from build123d import *

# Parameters (mm, degrees)
F1_DEPTH = 40
F2_DEPTH = 46
F4_DEPTH = 27
F5_DEPTH = 60.6


with BuildPart() as f1:
    # F0 (on Top) → F1 (new body, symmetric)
    with BuildSketch(Plane.XY):
        with BuildLine():
            Line((-49, 0), (0, 0))
            Line((0, 0), (41, 0))
            Line((41, 0), (41, 10))
            Line((41, 10), (42.9, 10))
            Line((42.9, 10), (49, 10))
            ThreePointArc((49, 10), (43.3431457505, 12.3431457505), (41, 18))
            Line((41, 18), (41, 19.9))
            Line((41, 19.9), (0, 19.9))
            Line((0, 19.9), (-41, 19.9))
            Line((-41, 19.9), (-41, 18))
            ThreePointArc((-41, 18), (-43.3431457505, 12.3431457505), (-49, 10))
            Line((-49, 10), (-49, 9.95))
            Line((-49, 9.95), (-49, 0))
        make_face()
        Polygon((41, 0), (0, 0), (-49, 0), (-49, -15), (0, -15), (41, -15), align=None)
        with BuildLine():
            Line((41, 10), (41, 0))
            Line((41, 0), (41, -15))
            Line((41, -15), (63.5, -15))
            ThreePointArc((63.5, -15), (51, -2.5), (63.5, 10))
            Line((63.5, 10), (49, 10))
            Line((49, 10), (42.9, 10))
            Line((42.9, 10), (41, 10))
        make_face()
        with BuildLine():
            ThreePointArc((76, -2.5), (72.3388347648, -11.3388347648), (63.5, -15))
            Line((63.5, -15), (86, -15))
            Line((86, -15), (86, -2.5))
            Line((86, -2.5), (86, 10))
            Line((86, 10), (63.5, 10))
            ThreePointArc((63.5, 10), (72.3388347648, 6.3388347648), (76, -2.5))
        make_face()
        Polygon((86, -2.5), (86, -15), (131, -15), (131, 10), (86, 10), align=None)
        with BuildLine():
            Line((63.5, -2.5), (63.5, -13.5))
            ThreePointArc((63.5, -13.5), (71.2781745931, -10.2781745931), (74.5, -2.5))
            ThreePointArc((74.5, -2.5), (71.2781745931, 5.2781745931), (63.5, 8.5))
            Line((63.5, 8.5), (63.5, -2.5))
        make_face()
        with BuildLine():
            ThreePointArc((63.5, 8.5), (52.5, -2.5), (63.5, -13.5))
            Line((63.5, -13.5), (63.5, -2.5))
            Line((63.5, -2.5), (63.5, 8.5))
        make_face()
        with BuildLine():
            ThreePointArc((63.5, 10), (51, -2.5), (63.5, -15))
            Line((63.5, -15), (63.5, -13.5))
            ThreePointArc((63.5, -13.5), (52.5, -2.5), (63.5, 8.5))
            Line((63.5, 8.5), (63.5, 10))
        make_face()
        with BuildLine():
            Line((63.5, -13.5), (63.5, -15))
            ThreePointArc((63.5, -15), (72.3388347648, -11.3388347648), (76, -2.5))
            ThreePointArc((76, -2.5), (72.3388347648, 6.3388347648), (63.5, 10))
            Line((63.5, 10), (63.5, 8.5))
            ThreePointArc((63.5, 8.5), (71.2781745931, 5.2781745931), (74.5, -2.5))
            ThreePointArc((74.5, -2.5), (71.2781745931, -10.2781745931), (63.5, -13.5))
        make_face()
    extrude(amount=F1_DEPTH, both=True)

    # F0 (on Top) → F2 (join)
    with BuildSketch(Plane.XY):
        with BuildLine():
            ThreePointArc((63.5, 10), (51, -2.5), (63.5, -15))
            Line((63.5, -15), (63.5, -13.5))
            ThreePointArc((63.5, -13.5), (52.5, -2.5), (63.5, 8.5))
            Line((63.5, 8.5), (63.5, 10))
        make_face()
        with BuildLine():
            Line((63.5, -13.5), (63.5, -15))
            ThreePointArc((63.5, -15), (72.3388347648, -11.3388347648), (76, -2.5))
            ThreePointArc((76, -2.5), (72.3388347648, 6.3388347648), (63.5, 10))
            Line((63.5, 10), (63.5, 8.5))
            ThreePointArc((63.5, 8.5), (71.2781745931, 5.2781745931), (74.5, -2.5))
            ThreePointArc((74.5, -2.5), (71.2781745931, -10.2781745931), (63.5, -13.5))
        make_face()
    extrude(amount=F2_DEPTH)

    # F3 (on face) → F4 (cut)
    with BuildSketch(Plane(origin=(0, 19.9, 0), x_dir=(-1, 0, 0), z_dir=(0, 1, 0))):
        Polygon((-33, 0), (-28, 0), (-28, 28), (0, 28), (0, 33), (-33, 33), align=None)
        Polygon((28, 28), (28, 0), (28, -28), (0, -28), (-28, -28), (-28, 0), (-33, 0), (-33, -33), (0, -33), (33, -33), (33, 0), (33, 33), (0, 33), (0, 28), align=None)
    extrude(amount=-F4_DEPTH, mode=Mode.SUBTRACT)

    # F5 (cut): a face of the model
    f5_faces = [f1.faces().sort_by_distance(p)[0] for p in [
        (0, 19.9, 0),
    ]]
    extrude(f5_faces, amount=-F5_DEPTH, mode=Mode.SUBTRACT)


solid = f1.part
Part model, mm, in its own coordinate system. A direction names the side the tool comes from. Round coordinates to 2 decimals unless told otherwise and drop trailing zeros. Write each loop counter-clockwise with the first axis right and the second up, starting at its lowest first coordinate (ties: lowest second). Pieces come first, ordered by that corner, then holes. Notation, with made-up numbers: (21.5, 61.5) - (38.5, 61.5) arc R21 ccw to (38.5, 83.5) - close; hole circle Ø2 at (32.5, 0). An arc over 180 degrees is marked (long way). Use CSV: the item, a comma, the result in double quotes.
Item 1: Flat gauge pins, fed straight in: P1, Ø2, axis at x = 93.5, z = -31, coming from the +Y side; P2, Ø8, axis at y = 13, z = -9.5, coming from the -X side; P3, Ø7.5, axis at x = 100.5, y = -8.5, coming from the +Z side; P4, Ø0.6, axis at y = 19, z = 9.5, coming from the +X side. Where does each tip first touch, or does it go through?
Results list:
P1,"stops at y = 10"
P2,"stops at x = -49"
P3,"stops at z = 40"
P4,"stops at x = 41"
Item 2: Slice it at B-B, the plane y = -10.5. Write the cut outline in (x, z), then the cut area to 3 significant figures.
Results list:
outline,"(-49, -40) - (131, -40) - (131, 40) - (73.1, 40) - (73.1, 46) - (71.05, 46) - (71.05, 40) - (55.95, 40) - (55.95, 46) - (53.9, 46) - (53.9, 40) - (-49, 40) - close; hole (-28, -28) - (28, -28) - (28, 28) - (-28, 28) - close"
area,"11,300 mm²"
Item 3: Wall check: L1, parallel to X at y = -12.5, z = 10.5; L2, parallel to Z at x = 8, y = 7; L3, parallel to X at y = 1, z = -5. Give the ranges that are in metal, low to high.
Results list:
L1,"x = -49 to -28, 28 to 131"
L2,"z = -40 to -33, 33 to 40"
L3,"x = -49 to -33, 33 to 131"
Item 4: Slice it at A-A, the plane z = -12. Write the cut outline in (x, y).
Results list:
outline,"(-49, -15) - (-28, -15) - (-28, -7.1) - (-33, -7.1) - (-33, 19.9) - (-41, 19.9) - (-41, 18) arc R8 cw to (-49, 10) - close; (28, -15) - (131, -15) - (131, 10) - (49, 10) arc R8 cw to (41, 18) - (41, 19.9) - (33, 19.9) - (33, -7.1) - (28, -7.1) - close"
Item 5: Slice it at C-C, the plane x = 103.5. Write the cut outline in (y, z), then the cut area to 3 significant figures.
Results list:
outline,"(-15, -40) - (10, -40) - (10, 40) - (-15, 40) - close"
area,"2,000 mm²"
Item 6: Slice it at D-D, the plane y = 4.5. Write the cut outline in (x, z), then the cut area to 3 significant figures.
Results list:
outline,"(-49, -40) - (131, -40) - (131, 40) - (73.86, 40) - (73.86, 46) - (71.99, 46) - (71.99, 40) - (55.01, 40) - (55.01, 46) - (53.14, 46) - (53.14, 40) - (-49, 40) - close; hole (-33, -33) - (33, -33) - (33, 33) - (-33, 33) - close"
area,"10,100 mm²"
Item 7: Pull direction Z, two halves, no side cores. Call faces 1 (the flat face through (1, 19.9, -35)), 2 (the flat face through (104, -2, 40)), 3 (the flat face through (0, -11, 28)): pulls with the +Z half, pulls with the -Z half, needs draft (parallel to the pull), parting line crosses it, or undercut.
Results list:
face 1,"needs draft"
face 2,"pulls with the +Z half"
face 3,"undercut"
Item 8: Tool access for faces 4 (the flat face through (0, -11, -28)), 5 (the flat face through (-49, -2, 1)), 6 (the flat face through (91, 10, 1)), 7 (the flat face through (63, -2, 40)), 8 (the flat face through (0, 7, -33)): list every direction of +Z, -Z, +X, -X, +Y, -Y with a clear straight run to the whole face (end or side of a thin tool).
Results list:
face 4,"+Y, -Y"
face 5,"+Z, -Z, -X, +Y, -Y"
face 6,"+Z, -Z, +X, +Y"
face 7,"+Z"
face 8,"+Y"
